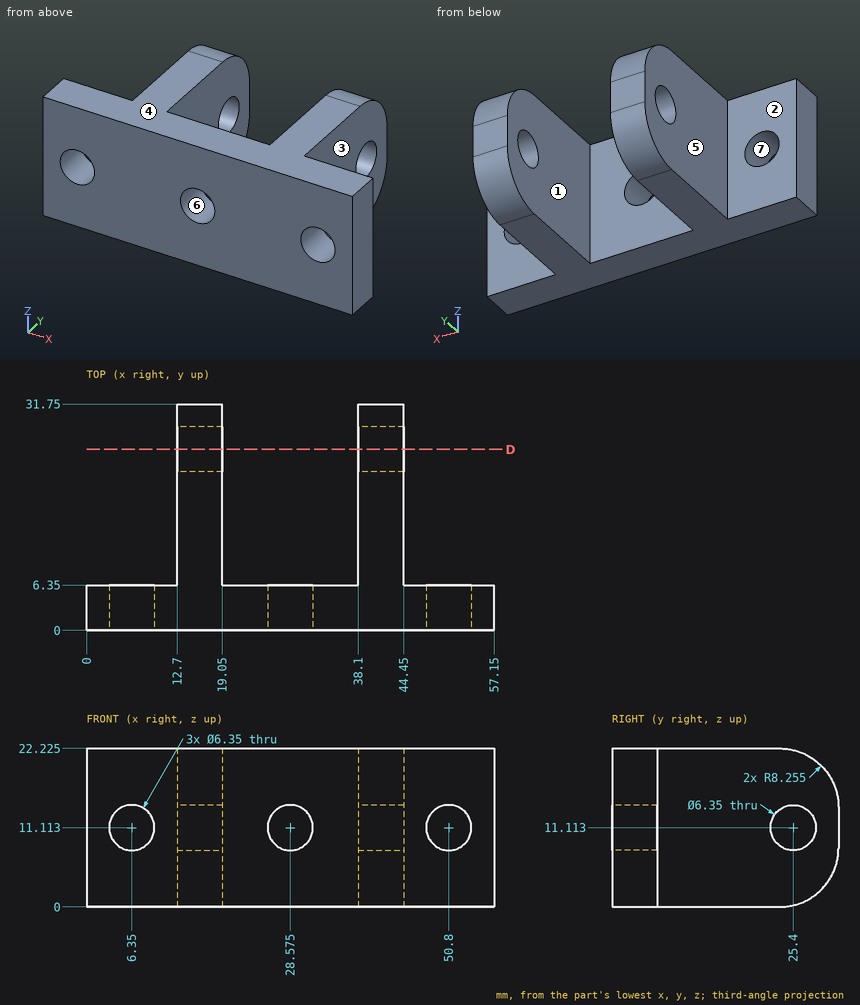
Part print with two shaded views. Sizes in mm from the minimum x, y, z corner. A direction names the side the tool comes from. Round coordinates to 2 decimals unless told otherwise and drop trailing zeros. Order: outer loops, then holes, each group sorted by start corner. A loop starts at its lowest first (then second) coordinate and runs counter-clockwise, first axis right, second up. Notation, with made-up numbers: M 21.25,43.25 L 44.25,43.25 A28 ccw 44.25,66.25 Z; hole C -30,57.25 d9. An arc over 180 degrees is marked long. Use CSV: the item, a comma, the result in double quotes.
Item 1: Probe probe 1 along X at (y, z) = (28, 3.5); probe 2 along Y at (x, z) = (52, 15.75); probe 3 along X at (y, z) = (2.5, 11.5). List the from-to ranges inside material, lowest first.
Worked answers:
probe 1,"12.7 to 19.05, 38.1 to 44.45"
probe 2,"0 to 6.35"
probe 3,"0 to 3.2, 9.5 to 25.42, 31.73 to 47.65, 53.95 to 57.15"
Item 2: Pull direction Z, two halves, no side cores. Call the marked faces 4, 5, 6 and 7: released by +Z, released by -Z, zero draft, split by the parting line, or undercut.
Worked answers:
face 4,"released by +Z"
face 5,"zero draft"
face 6,"undercut"
face 7,"undercut"
Item 3: Pin check, flat tips, straight feed: pin 1 (1.5 mm diameter, centred on x = 20.5, z = 12.5, fed in from -Y); pin 2 (10 mm diameter, centred on x = 8, z = 16.5, fed in from +Y); pin 3 (8.5 mm diameter, centred on y = 25.4, z = 11.11, fed in from +X); pin 4 (6.5 mm diameter, centred on y = 18.5, z = 13.5, fed in from -X). Stop position of each tip, or through.
Worked answers:
pin 1,"y = 0"
pin 2,"y = 31.71"
pin 3,"x = 44.45"
pin 4,"x = 12.7"
Item 4: Saw through at D-D (y = 25.4). List the corners of the cut face in (x, z).
Worked answers:
outline,"M 12.7,0.22 L 19.05,0.22 L 19.05,7.94 L 12.7,7.94 Z; M 12.7,14.29 L 19.05,14.29 L 19.05,22 L 12.7,22 Z; M 38.1,0.22 L 44.45,0.22 L 44.45,7.94 L 38.1,7.94 Z; M 38.1,14.29 L 44.45,14.29 L 44.45,22 L 38.1,22 Z"
Item 5: Which spindle directions (+Z, -Z, +X, -X, +Y, -Y) get a long thin tool onto all of the face, cutting with end or side? Do the marked faces 1, 2 and 3. Say none if no direction does.
Worked answers:
face 1,"+Z, -Z, +Y"
face 2,"+Z, -Z, -X, +Y"
face 3,"+Z, -Z, +X, +Y"
